Source: three-view drawing plus pictorial views. Frame: mm from the lowest corner of the part. A direction names the side the tool comes from. Give positions to 0.01 mm unless a question says otherwise; leave off trailing zeros. Write each loop counter-clockwise with the first axis right and the second up, starting at its lowest first coordinate (ties: lowest second). Pieces come first, ordered by that corner, then holes.
Q1. Cut plane A-A on z = 12.5. Return the cut outline in (x, y) (3 decimals).
Q2. Cut plane C-C on y = 8.75. Return the cut outline in (x, z) (3 decimals).
Q3. Pin query (flat end, axial travel): pin 1 (12 mm diameter, centred on x = 57, z = 19, fed in from +Y); pin 2 (3 mm diameter, centred on y = 9.5, z = 11.5, fed in from -X); pin 3 (4 mm diameter, centred on y = 12, z = 9.5, fed in from -X). Return the tip coordinate at first contact, or that it passes through.
Q4. Line query: L1, parallel to X at y = 7.25, z = 22.5; L2, parallel to Y at x = 67, z = 20.25; L3, parallel to Z at x = 37, y = 15 (3 decimals). Output: solid intervals per line, ascending.
Q5. Draft query along Y for the marked faces 1, 2, 3 and 4. Return one class per face: pulls with the +Y half, pulls with the -Y half, needs draft (parallel to the pull), parting line crosses it, or undercut.
Q6. Cut plane B-B on x = 31.5. Return the cut outline in (y, z), plus the area to 3 significant figures.
Q7. Cut plane D-D on x = 68.5. Return the cut outline in (y, z), plus the area to 3 significant figures.
Q8. Reachability of the marked faces 5 and 6 from +Z, -Z, +X, -X, +Y, -Y: full face, straight path, thin tool, end or side. Return the list, or none.
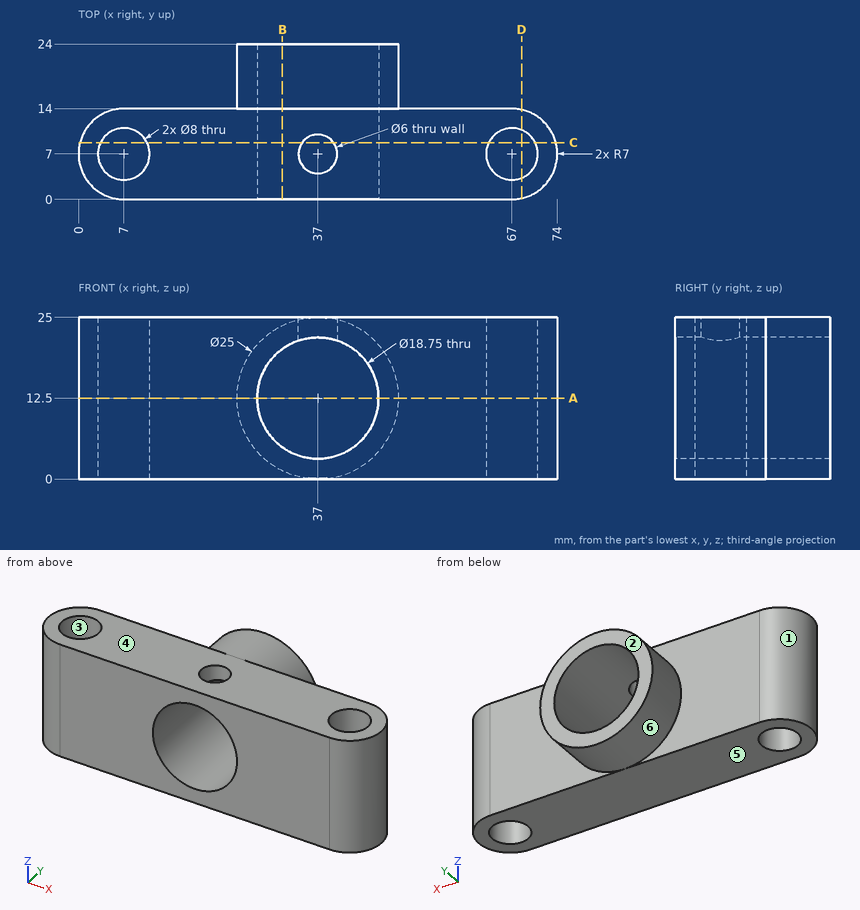
Data:
1. outline: (7, 0) - (27.625, 0) - (27.625, 24) - (24.5, 24) - (24.5, 14) - (7, 14) arc R7 ccw to start; (46.375, 0) - (67, 0) arc R7 ccw to (67, 14) - (49.5, 14) - (49.5, 24) - (46.375, 24) - close; hole circle Ø8 at (7, 7); hole circle Ø8 at (67, 7)
2. outline: (0.222, 0) - (3.403, 0) - (3.403, 25) - (0.222, 25) - close; (10.597, 0) - (63.403, 0) - (63.403, 25) - (39.437, 25) - (39.437, 21.553) arc R9.375 cw (long way) to (34.563, 21.553) - (34.563, 25) - (10.597, 25) - close; (70.597, 0) - (73.778, 0) - (73.778, 25) - (70.597, 25) - close
3. pin 1: stops at y = 14
3. pin 2: stops at x = 0.07
3. pin 3: stops at x = 0.68
4. L1: x = 0 to 3.01, 10.99 to 34.01, 39.99 to 63.01, 70.99 to 74
4. L2: y = 0 to 3, 11 to 14
4. L3: z = 0 to 3.125, 21.875 to 25
5. face 1: parting line crosses it
5. face 2: pulls with the +Y half
5. face 3: undercut
5. face 4: needs draft
6. outline: (0, 0) - (14, 0) - (14, 1.28) - (24, 1.28) - (24, 4.91) - (0, 4.91) - close; (0, 20.09) - (24, 20.09) - (24, 23.72) - (14, 23.72) - (14, 25) - (0, 25) - close
6. area: 210 mm2
7. outline: (0.16, 0) - (3.29, 0) - (3.29, 25) - (0.16, 25) - close; (10.71, 0) - (13.84, 0) - (13.84, 25) - (10.71, 25) - close
7. area: 156 mm2
8. face 5: -Z, +X, -X, +Y, -Y
8. face 6: +Y
